```python
from build123d import *

# Parameters (mm, degrees)
SKETCH1_W           = 14.4
SKETCH1_H           = 14.4
BOSS_EXTRUDE1_DEPTH = 19.7
SKETCH3_R           = 2.375
BOSS_EXTRUDE2_DEPTH = 12
SKETCH4_R           = 2.375
BOSS_EXTRUDE3_DEPTH = 12
CHAMFER1_SIZE       = 0.3
CHAMFER2_SIZE       = 0.5
SCALE1_SCALE        = 0.49


with BuildPart() as part:
    # Sketch1 → Boss-Extrude1 (new body)
    with BuildSketch(Plane(origin=(0, 0, 0), x_dir=(1, 0, 0), z_dir=(0, 1, 0))):
        Rectangle(SKETCH1_W, SKETCH1_H)
    extrude(amount=BOSS_EXTRUDE1_DEPTH)

    # Sketch2 → Cut-Revolve1 (revolve, cut)
    with BuildSketch(Plane.XY, mode=Mode.PRIVATE) as cut_revolve1_sk:
        Polygon((-6.95, 19.7), (-16.09, 19.7), (-16.09, 0), (-6.95, 0), (-13.55, 3.810511777), (-13.55, 15.889488223), align=None)
    revolve(cut_revolve1_sk.sketch.rotate(Axis((0, 20.685, 0), (0, -1, 0)), 270), axis=Axis((0, 20.685, 0), (0, -1, 0)), mode=Mode.SUBTRACT)

    # Sketch3 → Boss-Extrude2 (add, symmetric)
    with BuildSketch(Plane.XY):
        with Locations(Location((0, 6.7, 0), (0, 0, 180))):
            Circle(SKETCH3_R)
    extrude(amount=BOSS_EXTRUDE2_DEPTH, both=True)

    # Sketch4 → Boss-Extrude3 (add, symmetric)
    with BuildSketch(Plane(origin=(0, 0, 0), x_dir=(0, 0, -1), z_dir=(1, 0, 0))):
        with Locations((0, 13)):
            Circle(SKETCH4_R)
    extrude(amount=BOSS_EXTRUDE3_DEPTH, both=True)

    # Chamfer1
    chamfer1_edges = [part.edges().sort_by_distance(p)[0] for p in [
        (2.375, 6.7, -12),
        (2.375, 6.7, 12),
        (-12, 13, 2.375),
        (12, 13, 2.375),
    ]]
    chamfer(chamfer1_edges, length=CHAMFER1_SIZE)

    # Chamfer2
    chamfer2_edges = [part.edges().sort_by_distance(p)[0] for p in [
        (7.2, 9.85, 7.2),
        (7.2, 9.85, -7.2),
        (-7.2, 9.85, 7.2),
        (-7.2, 9.85, -7.2),
    ]]
    chamfer(chamfer2_edges, length=CHAMFER2_SIZE)


with BuildPart() as part_1:
    # Scale1: scaled about (0, 9.85, 0)
    add(part.part.scale(SCALE1_SCALE).moved(Location((0, 5.0235, 0))))


solid = part_1.part
```
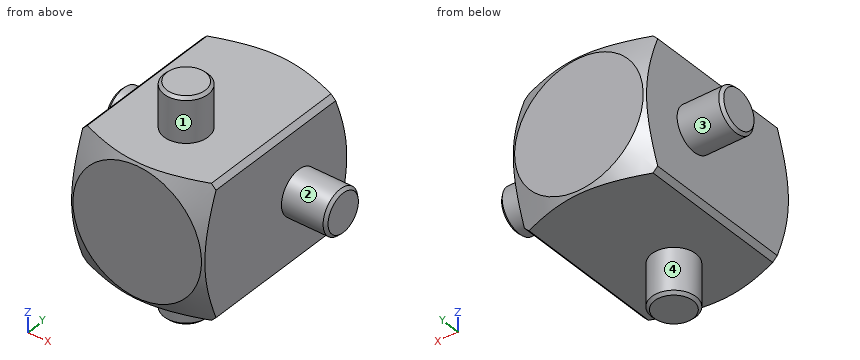
Work out the finished part from the listing and answer in its coordinate system (mm). Face numbers are marked on the shaded views. A direction names the side the tool comes from. Give positions to 0.01 mm unless a question says otherwise; leave off trailing zeros. Write each loop counter-clockwise with the first axis right and the second up, starting at its lowest first coordinate (ties: lowest second). Pieces come first, ordered by that corner, then holes.
(1) The part is cut by section A-A on x = 0. Write down the section's boundary in (y, z), plus the area to 3 significant figures.
Final values:
outline: (5.02, -3.41) - (5.09, -3.53) - (7.14, -3.53) - (7.14, -5.73) - (7.29, -5.88) - (9.32, -5.88) - (9.47, -5.73) - (9.47, -3.53) - (14.61, -3.53) - (14.68, -3.41) - (14.68, 3.41) - (14.61, 3.53) - (9.47, 3.53) - (9.47, 5.73) - (9.32, 5.88) - (7.29, 5.88) - (7.14, 5.73) - (7.14, 3.53) - (5.09, 3.53) - (5.02, 3.41) - close
area: 79.0 mm2
(2) A flat-ended cylindrical pin translates along its axis: pin 1 Ø5 at (x, y) = (1.5, 13.5) entering from +Z. Find the tip coordinate at first contact, or state that the pin passes through.
Final values:
pin 1: stops at z = 3.53
(3) The part is cut by section C-C on y = 10. Write down the section's boundary in (x, z).
Final values:
outline: (-3.53, -3.28) - (-3.28, -3.53) - (3.28, -3.53) - (3.53, -3.28) - (3.53, 3.28) - (3.28, 3.53) - (-3.28, 3.53) - (-3.53, 3.28) - close
(4) The part is cut by section D-D on y = 5.5. Write down the section's boundary in (x, z).
Final values:
outline: (-3.53, -2.34) arc R4.23 ccw to (-2.34, -3.53) - (2.34, -3.53) arc R4.23 ccw to (3.53, -2.34) - (3.53, 2.34) arc R4.23 ccw to (2.34, 3.53) - (-2.34, 3.53) arc R4.23 ccw to (-3.53, 2.34) - close
(5) The part is cut by section B-B on z = 0. Write down the section's boundary in (x, y).
Final values:
outline: (-5.88, 10.38) - (-5.73, 10.23) - (-3.53, 10.23) - (-3.53, 5.09) - (-3.41, 5.02) - (3.41, 5.02) - (3.53, 5.09) - (3.53, 10.23) - (5.73, 10.23) - (5.88, 10.38) - (5.88, 12.41) - (5.73, 12.56) - (3.53, 12.56) - (3.53, 14.61) - (3.41, 14.68) - (-3.41, 14.68) - (-3.53, 14.61) - (-3.53, 12.56) - (-5.73, 12.56) - (-5.88, 12.41) - close
(6) Straight lines are drawn through the part: line 1 (X direction, y = 9.5, z = -2); line 2 (Y direction, x = 5.5, z = 0). For each, find the intervals that lie inside material, in ascending order.
Final values:
line 1: x = -3.53 to 3.53
line 2: y = 10.23 to 12.56
(7) Which of the six approach directions +Z, -Z, +X, -X, +Y, -Y give full straight-line access (tool end or side, diameter ignored) to the marked faces 1, 2, 3 and 4?
Final values:
face 1: +Z
face 2: +X
face 3: -X
face 4: -Z
